Autodesk Inventor part; units mm, degrees
ref_plane "YZ Plane" through (0, 0, 0) normal (1, 0, 0) x (0, 1, 0)
ref_plane "XZ Plane" through (0, 0, 0) normal (0, 1, 0) x (-1, 0, 0)
ref_plane "XY Plane" through (0, 0, 0) normal (0, 0, 1) x (1, 0, 0)
sketch "スケッチ1" plane through (0, 0, 0) normal (1, 0, 0) x (0, 1, 0)
  line L0 (0, 0) -> (3.4, 0)
  line L1 (3.4, 0) -> (3.4, -83.525)
  line L2 (3.4, -83.525) -> (0, -83.525)
  line L3 (0, -83.525) -> (0, 0)
  line L4 (-6, 0) -> (-26, 0)
  line L5 (-26, 0) -> (-26, -134.3533)
  line L6 (-26, -134.3533) -> (-6, -134.3533)
  line L7 (-6, -134.3533) -> (-6, 0)
  line L8 (3.4, -83.525) -> (8.4, -83.525)
  line L9 (8.4, -83.525) -> (8.4, -73.125)
  line L10 (8.4, -73.125) -> (3.4, -73.125)
  line L11 (3.4, -73.125) -> (3.4, -83.525)
  line L12 (0, -73.125) -> (-26, -73.125)
  line L13 (-26, -73.125) -> (-26, -88.125)
  line L14 (-26, -88.125) -> (0, -88.125)
  line L15 (0, -88.125) -> (0, -73.125)
  line L16 (8.4, -83.525) -> (0, -83.525)
  line L17 (0, -83.525) -> (0, -88.125)
  line L18 (0, -88.125) -> (8.4, -88.125)
  line L19 (8.4, -88.125) -> (8.4, -83.525)
  circle A0 centre (-16, -76.625) radius 1.7
  circle A1 centre (-16, -84.625) radius 1.7
  point P0 (4.2, -88.125)
  point P1 (5.9, -83.525)
  point P2 (-26, -80.625)
  point P3 (3.4, -73.125)
  point P4 (-26, -73.125)
  dimension "d0" = 3.4
  dimension "d1" = 20
  dimension "d2" = 6
  dimension "d3" = 5
  dimension "d4" = 10.4
  dimension "d5" = 4.6
  dimension "d6" = 3.4
  dimension "d7" = 3.4
  dimension "d8" = 10
  dimension "d9" = 10
  dimension "d10" = 8
  dimension "d11" = 3.5
  dimension "d14" = 0
extrude "押し出し1" add sketch "スケッチ1" against normal blind 10 contours L3 L15 L14 L7 L12 | L10 L9 L8 L1 | L2 L8 L19 L18 L15 | L7 L14 L5 L12
fillet "フィレット1" radius 2 6 edges at (-5, 8.4, -73.125) (-5, 3.4, -73.125) (-5, 0, -73.125) (-5, -26, -73.125) (-5, -26, -88.125) (-5, 8.4, -88.125)
properties part number "base_weel-v2-3DP-C-F-2" material "ABS プラスチック"
For this review, take the finished solid that the model builds, in its own axes (mm). A direction names the side the tool comes from. Coordinates: 2 decimals unless noted, no trailing zeros. Write each loop counter-clockwise with the first axis right and the second up, starting at its lowest first coordinate (ties: lowest second). Pieces come first, ordered by that corner, then holes. Notation, with made-up numbers: (27.5, -13.75) - (45.5, -13.75) arc R20 ccw to (45.5, 16.25) - close; hole circle Ø2 at (-31, 56). An arc over 180 degrees is marked (long way). Put each result on its own line as item: value.
1. Add section B-B, the plane y = -16. Give the boundary of the cut face in (x, z) (3 decimals).
Values found:
outline: (-10, -88.125) - (0, -88.125) - (0, -86.325) - (-10, -86.325) - close; (-10, -82.925) - (0, -82.925) - (0, -78.325) - (-10, -78.325) - close; (-10, -74.925) - (0, -74.925) - (0, -73.125) - (-10, -73.125) - close
2. Add section D-D, the plane x = -1.5. Give the boundary of the cut face in (y, z) (3 decimals), then the cut area to 3 significant figures.
Values found:
outline: (-26, -86.125) arc R2 ccw to (-24, -88.125) - (6.4, -88.125) arc R2 ccw to (8.4, -86.125) - (8.4, -75.125) arc R2 ccw to (6.4, -73.125) - (5.4, -73.125) arc R2 ccw to (3.4, -75.125) - (3.4, -83.525) - (0, -83.525) - (0, -75.125) arc R2 ccw to (-2, -73.125) - (-24, -73.125) arc R2 ccw to (-26, -75.125) - close; hole circle Ø3.4 at (-16, -84.625); hole circle Ø3.4 at (-16, -76.625)
area: 457 mm²
3. Machinability: for faces 1 (the cylindrical face through (-5, -15, -78)), 2 (the cylindrical face through (-5.07, 3.97, -73.726)), which of the approach directions +Z, -Z, +X, -X, +Y, -Y give a long, thin tool a straight path to every point of the face, cutting with its end or side? Answer none if there is none.
Values found:
face 1: +X, -X
face 2: +Z, +X, -X
4. Add section C-C, the plane z = -77.25. Give the boundary of the cut face in (x, y).
Values found:
outline: (-10, -26) - (0, -26) - (0, -17.58) - (-10, -17.58) - close; (-10, -14.42) - (0, -14.42) - (0, 0) - (-10, 0) - close; (-10, 3.4) - (0, 3.4) - (0, 8.4) - (-10, 8.4) - close
5. Add section A-A, the plane z = -79.25. Give the boundary of the cut face in (x, y).
Values found:
outline: (-10, -26) - (0, -26) - (0, 0) - (-10, 0) - close; (-10, 3.4) - (0, 3.4) - (0, 8.4) - (-10, 8.4) - close
6. For pin 1 (2 mm diameter, centred on y = -16, z = -76.625, fed in from +X); pin 2 (3.5 mm diameter, centred on x = -6, y = 1.5, fed in from +Z), all flat-tipped, find the tip position at first contact; note any pin that passes through.
Values found:
pin 1: through
pin 2: z = -74.16
7. Mouldability with a two-part tool opening along Y and no side actions: class faces 3 (the flat face through (-5, 3.4, -79)), 4 (the flat face through (-5, 8.4, -81)), 5 (the flat face through (-5, -13, -73.125)) as released by +Y, released by -Y, zero draft, split by the parting line, or undercut.
Values found:
face 3: undercut
face 4: released by +Y
face 5: zero draft
8. Wall thickness on probe 1 along Z at (x, y) = (-7.25, -16) (3 decimals); probe 2 along Y at (x, z) = (-5.5, -79.5); probe 3 along Y at (x, z) = (-6, -78): over which ranges is each line inside the solid? List them lowest first.
Values found:
probe 1: -88.125 to -86.325, -82.925 to -78.325, -74.925 to -73.125
probe 2: -26 to 0, 3.4 to 8.4
probe 3: -26 to -17, -15 to 0, 3.4 to 8.4
